from build123d import *

# Parameters (mm, degrees)
CROQUIS1_R              = 2.5
SALIENTE_EXTRUIR1_DEPTH = 2
SALIENTE_EXTRUIR2_DEPTH = 0.2
PATR_N_START            = -2
PATR_N_DE_RAYADO2_DEPTH = 4.2


# Read off the part's stored shape, not the designer's step: Patrón de rayado2
with BuildPart() as part:
    # Croquis1 → Saliente-Extruir1 (new, symmetric)
    with BuildSketch(Plane(origin=(0, 0, 0), x_dir=(1, 0, 0), z_dir=(0, 1, 0))):
        with BuildLine():
            Line((0, 7.25), (55, 5))
            ThreePointArc((55, 5), (60, 0), (55, -5))
            Line((55, -5), (0, -7.25))
            ThreePointArc((0, -7.25), (-7.25, 0), (0, 7.25))
        make_face()
        with Locations(Location((0, 0, 0), (0, 0, 270))):
            Circle(CROQUIS1_R, mode=Mode.SUBTRACT)
        with Locations(Location((55, 0, 0), (0, 0, 270))):
            Circle(CROQUIS1_R, mode=Mode.SUBTRACT)
    extrude(amount=SALIENTE_EXTRUIR1_DEPTH, both=True)

    # Croquis2 → Saliente-Extruir2 (add)
    with BuildSketch(Plane(origin=(0, 2, 0), x_dir=(1, 0, 0), z_dir=(0, 1, 0))):
        with BuildLine():
            Line((7, 4.880145328), (7, -4.880145328))
            ThreePointArc((7, -4.880145328), (7.614990904, -6.322972346), (9.081749804, -6.878473872))
            Line((9.081749804, -6.878473872), (43.081749804, -5.487564781))
            ThreePointArc((43.081749804, -5.487564781), (44.442827018, -4.874245333), (45, -3.489236237))
            Line((45, -3.489236237), (45, 3.489236237))
            ThreePointArc((45, 3.489236237), (44.442827018, 4.874245333), (43.081749804, 5.487564781))
            Line((43.081749804, 5.487564781), (9.081749804, 6.878473872))
            ThreePointArc((9.081749804, 6.878473872), (7.614990904, 6.322972346), (7, 4.880145328))
        make_face()
    extrude(amount=SALIENTE_EXTRUIR2_DEPTH)

    # Patrón de rayado2 outline → Patrón de rayado2 (cut)
    with BuildSketch(Plane(origin=(0, 0, 0), x_dir=(1, 0, 0), z_dir=(0, 1, 0)).offset(PATR_N_START)):
        Polygon((10.504788453, 2.748868179), (11.433155318, 0.977389992), (13.431483862, 0.895640188), (14.501445541, 2.585368571), (13.573078676, 4.356846757), (11.574750132, 4.438596561), align=None)
        Polygon((20.48865892, 0.606937572), (22.486987464, 0.525187768), (23.556949143, 2.21491615), (22.628582278, 3.986394337), (20.630253734, 4.068144141), (19.560292055, 2.378415759), align=None)
        Polygon((29.544162522, 0.236485152), (31.542491066, 0.154735348), (32.612452745, 1.84446373), (31.68408588, 3.615941917), (29.685757336, 3.697691721), (28.615795657, 2.007963338), align=None)
        Polygon((38.599666124, -0.133967268), (40.597994668, -0.215717072), (41.667956347, 1.47401131), (40.739589483, 3.245489496), (38.741260939, 3.327239301), (37.67129926, 1.637510918), align=None)
        Polygon((19.387547255, -1.84423492), (20.31591412, -3.615713106), (22.314242664, -3.69746291), (23.384204343, -2.007734528), (22.455837478, -0.236256342), (20.457508934, -0.154506537), align=None)
        Polygon((11.260410517, -3.245260686), (13.258739061, -3.32701049), (14.32870074, -1.637282108), (13.400333876, 0.134196079), (11.402005332, 0.215945883), (10.332043653, -1.473782499), align=None)
        Polygon((33.057175058, -0.288588211), (33.985541923, -2.060066397), (35.983870467, -2.141816201), (37.053832146, -0.452087819), (36.125465281, 1.319390367), (34.127136737, 1.401140171), align=None)
        Polygon((24.930038321, -1.689613977), (26.928366865, -1.771363781), (27.998328544, -0.081635399), (27.069961679, 1.689842788), (25.071633135, 1.771592592), (24.001671456, 0.081864209), align=None)
        Polygon((15.874534719, -1.319161557), (17.872863263, -1.400911361), (18.942824942, 0.288817021), (18.014458077, 2.060295208), (16.016129533, 2.142045012), (14.946167854, 0.45231663), align=None)
    extrude(amount=PATR_N_DE_RAYADO2_DEPTH, mode=Mode.SUBTRACT)


solid = part.part
Could you check a few things on this model? Use its own coordinates, in mm. A direction names the side the tool comes from. Coordinates: 2 decimals unless noted, no trailing zeros. Order: outer loops, then holes, each group sorted by start corner. A loop starts at its lowest first (then second) coordinate and runs counter-clockwise, first axis right, second up.
Q1. Please list where these lines run through material, in increasing order: L1, parallel to X at y = -0.8, z = 3; L2, parallel to Z at x = 18, y = -0.8; L3, parallel to Z at x = 30, y = 1.75.
Q2. Which directions (+Z, -Z, +X, -X, +Y, -Y) give clear straight access to the entire face, cutting with the end or side of a thin tool? Please do faces 4 (the flat face through (12.415, 0.071, -0.174)), 5 (the flat face through (26, 2.2, 3)).
Q3. Suppose I cut it at A-A on x = 21.5. Please give me the cut outline in (y, z), and give its area (3 significant figures).
Q4. Suppose I cut it at B-B on y = 0.7. Give the number of separate pieces and of enclosed holes in the cut face, and give its area (3 significant figures).
Q5. Thinking about a two-plate mould opening in Z: for faces 1 (the flat face through (23.014, 0.071, -1.358)), 2 (the flat face through (52, 2, 0)), 3 (the cylindrical face through (-7.25, 0.03, 0.16)), which applies, released by +Z, released by -Z, zero draft, split by the parting line, or undercut?
Q6. Will these pins go through, and if not, where does the flat tip stop? pin 1 (3 mm diameter, centred on x = 47.5, z = -4, fed in from +Y); pin 2 (1 mm diameter, centred on x = 11.5, y = 1.5, fed in from -Z); pin 3 (1 mm diameter, centred on y = -0.5, z = 1.5, fed in from +X).
Q7. Suppose I cut it at C-C on x = 4. Please give me the cut outline in (y, z).
Answer:
1. L1: x = -6.6 to 11.13, 13.47 to 19.99, 22.76 to 59
1. L2: z = -6.51 to -2.06, 1.2 to 6.51
1. L3: z = -6.02 to -3.68, -0.22 to 6.02
2. face 4: +Y, -Y
2. face 5: +Z, -Z, +X, -X, +Y
3. outline: (-2, -6.37) - (2.2, -6.37) - (2.2, -4.03) - (-2, -4.03) - close; (-2, -0.57) - (2.2, -0.57) - (2.2, 0.2) - (-2, 0.2) - close; (-2, 3.66) - (2.2, 3.66) - (2.2, 6.37) - (-2, 6.37) - close
3. area: 24.4 mm2
4. separate pieces: 1
4. enclosed holes: 11
4. area: 663 mm2
5. face 1: undercut
5. face 2: zero draft
5. face 3: split by the parting line
6. pin 1: stops at y = 2
6. pin 2: stops at z = -6.8
6. pin 3: stops at x = 59.9
7. outline: (-2, -7.09) - (2, -7.09) - (2, 7.09) - (-2, 7.09) - close
